The model under review builds one solid part; all positions refer to its coordinate system, in mm. Coordinates: 2 decimals unless noted, no trailing zeros. Loops run counter-clockwise (first coordinate to the right, second up) from the corner with the lowest first, then second, coordinate; pieces in that order, holes last. Notation, with made-up numbers: M 31.5,-28.75 L 63.5,-28.75 A18 ccw 63.5,-16.75 Z; hole C -30.75,85 d2. An arc over 180 degrees is marked long. Return JSON: item names as keys, results as strings.
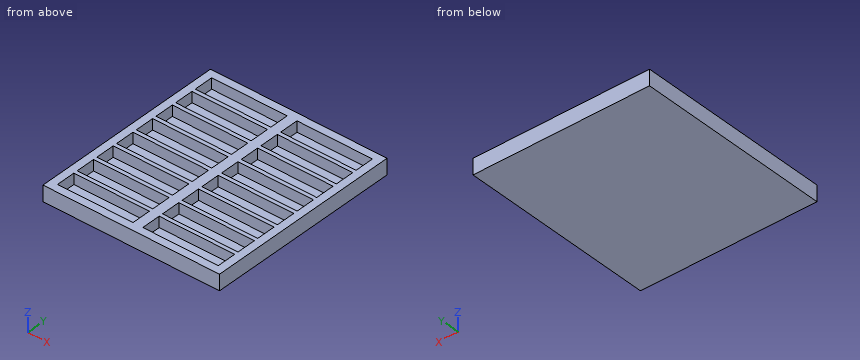
```python
from build123d import *

# Parameters (mm, degrees)
F0_W     = 180
F0_H     = 200
F1_DEPTH = 16
F2_W     = 77
F2_H     = 19.5
F3_DEPTH = 11


with BuildPart() as f1:
    # F0 (on Top) → F1 (new body)
    with BuildSketch(Plane.XY):
        Rectangle(F0_W, F0_H)
    extrude(amount=F1_DEPTH)

    # F2 (on face) → F3 (cut)
    with BuildSketch(Plane.XY.offset(16)):
        with Locations((-43.5, 82.25)):
            Rectangle(F2_W, F2_H)
        with Locations((-43.5, 58.75)):
            Rectangle(F2_W, F2_H)
        with Locations((43.5, 58.75)):
            Rectangle(F2_W, F2_H)
        with Locations((43.5, 82.25)):
            Rectangle(F2_W, F2_H)
        with Locations((43.5, 35.25)):
            Rectangle(F2_W, F2_H)
        with Locations((-43.5, 35.25)):
            Rectangle(F2_W, F2_H)
        with Locations((-43.5, 11.75)):
            Rectangle(F2_W, F2_H)
        with Locations((43.5, 11.75)):
            Rectangle(F2_W, F2_H)
        with Locations((43.5, -11.75)):
            Rectangle(F2_W, F2_H)
        with Locations((-43.5, -11.75)):
            Rectangle(F2_W, F2_H)
        with Locations((-43.5, -35.25)):
            Rectangle(F2_W, F2_H)
        with Locations((43.5, -35.25)):
            Rectangle(F2_W, F2_H)
        with Locations((-43.5, -58.75)):
            Rectangle(F2_W, F2_H)
        with Locations((43.5, -58.75)):
            Rectangle(F2_W, F2_H)
        with Locations((-43.5, -82.25)):
            Rectangle(F2_W, F2_H)
        with Locations((43.5, -82.25)):
            Rectangle(F2_W, F2_H)
    extrude(amount=-F3_DEPTH, mode=Mode.SUBTRACT)


solid = f1.part
```
1. To check wall thickness, follow line 1 (X direction, y = 85.5, z = 15.25); line 2 (Z direction, x = 79.5, y = -18). State the ranges of each line that lie inside material, in increasing order.
Check values:
{"line 1": "-90 to -82, -5 to 5, 82 to 90", "line 2": "0 to 5"}
2. Insertion check: pin 1 Ø5 at (x, y) = (28.5, 12.5) entering from +Z. The pin has a flat end and moves straight along its axis. Give the tip position at first contact, or say it passes through.
Check values:
{"pin 1": "z = 5"}
3. Add section B-B on z = 13. State how many separate pieces and enclosed holes the cut face has, plus the area to 3 significant figures.
Check values:
{"separate pieces": "1", "enclosed holes": "16", "area": "12,000 mm²"}
4. Add section A-A on y = 81. Give the boundary of the cut face in (x, z).
Check values:
{"outline": "M -90,0 L 90,0 L 90,16 L 82,16 L 82,5 L 5,5 L 5,16 L -5,16 L -5,5 L -82,5 L -82,16 L -90,16 Z"}
